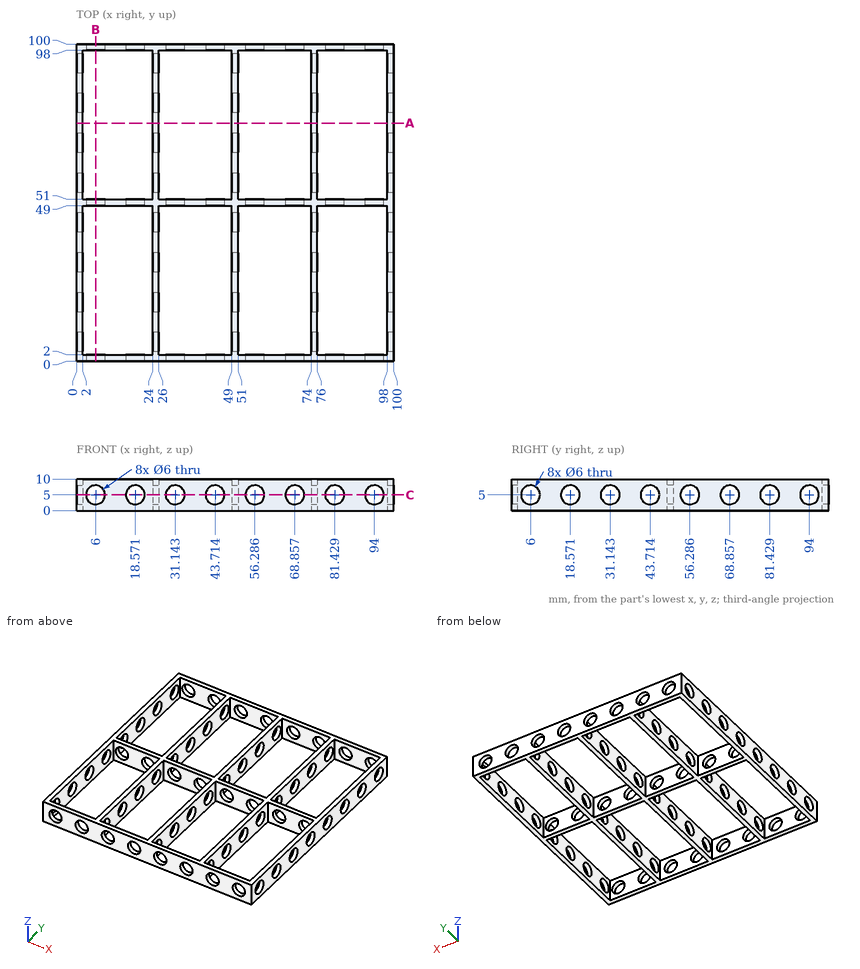
Study the drawing (mm; zero at the part's minimum x, y, z) and answer. Give positions to 0.01 mm unless a question says otherwise; leave off trailing zeros. Write each loop counter-clockwise with the first axis right and the second up, starting at its lowest first coordinate (ties: lowest second). Pieces come first, ordered by that corner, then holes. Notation, with made-up numbers: (6.25, 27.5) -> (13.25, 27.5) arc R25 ccw to (13.25, 40.5) -> close; hole circle Ø3 at (38.25, 13). An arc over 180 degrees is marked (long way). Write item = value, one per line.
Q1. A flat-ended cylindrical pin translates along its axis: pin 1 Ø2 at (y, z) = (72, 4.5) entering from -X. Find the tip coordinate at first contact, or state that the pin passes through.
Computed values:
pin_1 = 0
Q2. Consider line 1 along X through (y, z) = (96.5, 8.5); line 2 along Y through (x, z) = (13.5, 6.25); line 3 along Z through (x, y) = (6, 50). Determine where each line is inside the solid, lowest interval first.
Computed values:
line_1 = 0 to 2, 24 to 26, 49 to 51, 74 to 76, 98 to 100
line_2 = 0 to 2, 49 to 51, 98 to 100
line_3 = 0 to 2, 8 to 10
Q3. Section B-B on x = 6 is taken. Determine the outline of the cut face in (y, z), and give its area (3 significant figures).
Computed values:
outline = (0, 0) -> (2, 0) -> (2, 2) -> (0, 2) -> close; (0, 8) -> (2, 8) -> (2, 10) -> (0, 10) -> close; (49, 0) -> (51, 0) -> (51, 2) -> (49, 2) -> close; (49, 8) -> (51, 8) -> (51, 10) -> (49, 10) -> close; (98, 0) -> (100, 0) -> (100, 2) -> (98, 2) -> close; (98, 8) -> (100, 8) -> (100, 10) -> (98, 10) -> close
area = 24.0 mm^2
Q4. Section C-C on z = 5 is taken. State how many separate pieces and enclosed holes the cut face has.
Computed values:
separate_pieces = 57
enclosed_holes = 0
Q5. Section A-A on y = 75 is taken. Determine the outline of the cut face in (x, z), and give its area (3 significant figures).
Computed values:
outline = (0, 0) -> (2, 0) -> (2, 10) -> (0, 10) -> close; (24, 0) -> (26, 0) -> (26, 10) -> (24, 10) -> close; (49, 0) -> (51, 0) -> (51, 10) -> (49, 10) -> close; (74, 0) -> (76, 0) -> (76, 10) -> (74, 10) -> close; (98, 0) -> (100, 0) -> (100, 10) -> (98, 10) -> close
area = 100 mm^2
